```python
from build123d import *

# Parameters (mm, degrees)
BOSS_EXTRUDE1_DEPTH      = 457.2
BOSS_EXTRUDE1_DEPTH_BACK = 457.2
SKETCH3_W                = 76.2
SKETCH3_H                = 50.8
SKETCH3_W_2              = 69.85
SKETCH3_H_2              = 44.45
SKETCH6_R                = 6.394880264
SKETCH6_R_2              = 6.789577508
SKETCH6_R_3              = 5.5626
CUT_EXTRUDE1_DEPTH       = 462.588658873


with BuildPart() as part:
    # Sketch3 → Boss-Extrude1 (new, two sides: drawn at the far end of the back side and taken through both)
    with BuildSketch(Plane.XY.offset(-BOSS_EXTRUDE1_DEPTH_BACK)):
        Rectangle(SKETCH3_W, SKETCH3_H)
        Rectangle(SKETCH3_W_2, SKETCH3_H_2, mode=Mode.SUBTRACT)
    extrude(amount=BOSS_EXTRUDE1_DEPTH + BOSS_EXTRUDE1_DEPTH_BACK)

    # Sketch6 → Cut-Extrude1 (cut, through all)
    with BuildSketch(Plane(origin=(0, 25.4, 0), x_dir=(1, 0, 0), z_dir=(0, 1, 0))):
        with Locations(Location((-19.05, -228.6, 0), (0, 0, 270))):
            Circle(SKETCH6_R)
        with Locations(Location((19.05, -228.6, 0), (0, 0, 270))):
            Circle(SKETCH6_R_2)
        with Locations(Location((19.05, 228.6, 0), (0, 0, 270))):
            Circle(SKETCH6_R_2)
        with Locations(Location((-19.05, 228.6, 0), (0, 0, 270))):
            Circle(SKETCH6_R)
        with Locations(Location((0, -352.425, 0), (0, 0, 270))):
            Circle(SKETCH6_R_3)
        with Locations(Location((0, -409.575, 0), (0, 0, 270))):
            Circle(SKETCH6_R_3)
        with Locations(Location((0, 409.575, 0), (0, 0, 270))):
            Circle(SKETCH6_R_3)
        with Locations(Location((0, 352.425, 0), (0, 0, 270))):
            Circle(SKETCH6_R_3)
    extrude(amount=-CUT_EXTRUDE1_DEPTH, mode=Mode.SUBTRACT)


solid = part.part
```
Check sheet for the modelled part. Datum: model origin and axes. Units: mm. A direction names the side the tool comes from. Round coordinates to 2 decimals unless told otherwise and drop trailing zeros. Order: outer loops, then holes, each group sorted by start corner. A loop starts at its lowest first (then second) coordinate and runs counter-clockwise, first axis right, second up. Notation, with made-up numbers: (50.25, 29) -> (74.25, 29) arc R22 cw to (74.25, 59) -> close; hole circle Ø1 at (-23, 64.25). An arc over 180 degrees is marked (long way). Use CSV: the item, a comma, the result in double quotes.
(1) Material ranges on line 1 along X through (y, z) = (-24, 228); line 2 along X through (y, z) = (-5, 404) (3 decimals); line 3 along Y through (x, z) = (-26.5, -77.5) (3 decimals), recorded low to high. Write a range as from..to.
Worked out:
line 1,"-38.1..-25.42, -12.68..12.29, 25.81..38.1"
line 2,"-38.1..-34.925, 34.925..38.1"
line 3,"-25.4..-22.225, 22.225..25.4"
(2) Cross-section at A-A (y = 7.5). Record the boundary of the cut face in (x, z) (3 decimals).
Worked out:
outline,"(-38.1, -457.2) -> (-34.925, -457.2) -> (-34.925, 457.2) -> (-38.1, 457.2) -> close; (34.925, -457.2) -> (38.1, -457.2) -> (38.1, 457.2) -> (34.925, 457.2) -> close"
(3) Cross-section at B-B (z = 183.5). Record the boundary of the cut face in (x, y) (3 decimals).
Worked out:
outline,"(-38.1, -25.4) -> (38.1, -25.4) -> (38.1, 25.4) -> (-38.1, 25.4) -> close; hole (-34.925, -22.225) -> (34.925, -22.225) -> (34.925, 22.225) -> (-34.925, 22.225) -> close"
(4) Tool access check on faces 1 (the face through (-34.925, 0, -6)), 2 (the face through (-38.1, 0, -6)). Record the directions out of +Z, -Z, +X, -X, +Y, -Y that give a thin tool (end or side, any length) a straight path to the whole face; none if there is none.
Worked out:
face 1,"+Z, -Z"
face 2,"+Z, -Z, -X, +Y, -Y"
(5) Depth check by flat-ended pin: pin 1 (14.5 mm diameter, centred on x = -19.05, z = -228.6, fed in from +Y); pin 2 (9 mm diameter, centred on x = 0, z = -352.425, fed in from -Y). Enter the tip coordinate at first touch or a pass-through.
Worked out:
pin 1,"y = 25.4"
pin 2,"through"
(6) Draft check along Y on faces 3 (the face through (0, -22.225, -6)), 4 (the face through (-1, 25.4, -6)), 5 (the face through (-3, -22.5, 457.2)). Enter one of: pulls with the +Y half, pulls with the -Y half, needs draft (parallel to the pull), parting line crosses it, or undercut.
Worked out:
face 3,"undercut"
face 4,"pulls with the +Y half"
face 5,"needs draft"
